```python
from build123d import *

# Parameters (mm, degrees)
F1_DEPTH = 76.2
F3_D     = 19.05
F5_D     = 19.05


with BuildPart() as f1:
    # F0 (on Front) → F1 (new body)
    with BuildSketch(Plane.XZ):
        Polygon((-50.8, -75.233199), (-127, -75.233199), (-127, -126.033199), (0, -126.033199), (0, -103.410661), (-50.8, -103.410661), align=None)
    extrude(amount=F1_DEPTH)

    # F3 (through all)
    with Locations(Plane.YZ.offset(-50.8)):
        with Locations((-36.601152, -89.32193)):
            Hole(F3_D / 2)

    # F5 (through all)
    with Locations(Plane.XY.offset(-75.233199)):
        with Locations((-88.9, -38.1)):
            Hole(F5_D / 2)


solid = f1.part
```
Input: part model. Units: mm. Frame: model coordinates. A direction names the side the tool comes from. Coordinates: 2 decimals unless noted, no trailing zeros. Order: outer loops, then holes, each group sorted by start corner. A loop starts at its lowest first (then second) coordinate and runs counter-clockwise, first axis right, second up. Notation, with made-up numbers: (56.5, 36) - (95.5, 36) arc R23 ccw to (95.5, 68) - close; hole circle Ø8 at (-11, 49). An arc over 180 degrees is marked (long way). Put each result on its own line as item: value.
1. Draft query along Y for faces 1 (the face through (0, -38, -115)), 2 (the face through (-79, 0, -106)), 3 (the face through (-86.84, -47.4, -106.63)), 4 (the face through (-79, -76.2, -106)). Return one class per face: pulls with the +Y half, pulls with the -Y half, needs draft (parallel to the pull), parting line crosses it, or undercut.
Report:
face 1: needs draft
face 2: pulls with the +Y half
face 3: undercut
face 4: pulls with the -Y half
2. Reachability of faces 5 (the face through (-25, -38, -103.411)), 6 (the face through (-89.433, -27.085, -88.903)) from +Z, -Z, +X, -X, +Y, -Y: full face, straight path, thin tool, end or side. Return the list, or none.
Report:
face 5: +Z, +X, +Y, -Y
face 6: +X, -X
3. Cut plane B-B on z = -96. Return the cut outline in (x, y) (3 decimals).
Report:
outline: (-127, -76.2) - (-50.8, -76.2) - (-50.8, -43.393) - (-80.981, -43.393) arc R9.525 cw to (-96.819, -43.393) - (-127, -43.393) - close; (-127, -29.809) - (-93.589, -29.809) arc R9.525 cw to (-84.211, -29.809) - (-50.8, -29.809) - (-50.8, 0) - (-127, 0) - close
4. Cut plane A-A on y = -38.1. Return the cut outline in (x, z) (3 decimals).
Report:
outline: (-127, -126.033) - (-98.425, -126.033) - (-98.425, -98.728) - (-127, -98.728) - close; (-127, -79.916) - (-98.425, -79.916) - (-98.425, -75.233) - (-127, -75.233) - close; (-79.375, -126.033) - (0, -126.033) - (0, -103.411) - (-50.8, -103.411) - (-50.8, -98.728) - (-79.375, -98.728) - close; (-79.375, -79.916) - (-50.8, -79.916) - (-50.8, -75.233) - (-79.375, -75.233) - close
5. Line query: line 1 along Y through (x, z) = (-80, -89.5); line 2 along Y through (x, z) = (-88.9, -98.5) (3 decimals); line 3 along X through (y, z) = (-38, -115). Output: solid intervals per line, ascending.
Report:
line 1: y = -76.2 to -46.12, -27.08 to 0
line 2: y = -76.2 to -47.625, -28.575 to 0
line 3: x = -127 to -98.42, -79.38 to 0
6. Contact query for a flat-ended pin moving along its axis: pin 1 Ø10 at (y, z) = (-30, -82) entering from +X. Output: stop coordinate, or through.
Report:
pin 1: stops at x = -50.8
7. Cut plane D-D on z = -117. Return the cut outline in (x, y) (3 decimals), then the cut area to 3 significant figures.
Report:
outline: (-127, -76.2) - (0, -76.2) - (0, 0) - (-127, 0) - close; hole circle Ø19.05 at (-88.9, -38.1)
area: 9,390 mm2
8. Cut plane C-C on x = -88.9. Return the cut outline in (y, z) (3 decimals), then the cut area to 3 significant figures.
Report:
outline: (-76.2, -126.033) - (-47.625, -126.033) - (-47.625, -75.233) - (-76.2, -75.233) - close; (-28.575, -126.033) - (0, -126.033) - (0, -75.233) - (-28.575, -75.233) - (-28.575, -84.193) arc R9.525 cw to (-28.575, -94.451) - close
area: 2,890 mm2
